Here's how the part is built. I have some questions about the finished solid (model axes, mm). Round coordinates to 2 decimals unless told otherwise and drop trailing zeros. Order: outer loops, then holes, each group sorted by start corner. A loop starts at its lowest first (then second) coordinate and runs counter-clockwise, first axis right, second up. Notation, with made-up numbers: (9.5, 5) - (27.5, 5) arc R9 cw to (27.5, 18) - close; hole circle Ø11 at (-25.5, 57.5). An arc over 180 degrees is marked (long way). One line per item, written item: value.
Autodesk Inventor part; units mm, degrees
ref_plane "YZ Plane" through (0, 0, 0) normal (1, 0, 0) x (0, 1, 0)
ref_plane "XZ Plane" through (0, 0, 0) normal (0, 1, 0) x (-1, 0, 0)
ref_plane "XY Plane" through (0, 0, 0) normal (0, 0, 1) x (1, 0, 0)
sketch "Sketch1" plane through (0, 0, 0) normal (0, 0, 1) x (1, 0, 0)
  circle A0 centre (13.2036, 20.3187) radius 2.0955
  circle A1 centre (-12.1964, 20.3187) radius 2.0955
  line L0 (4.3471, -17.7813) -> (-3.3398, -17.7813)
  arc A2 (4.3471, -17.7813) -> (7.3873, -15.5216) centre (4.3471, -14.6063) ccw
  arc A3 (-6.38, -15.5216) -> (-3.3398, -17.7813) centre (-3.3398, -14.6063) ccw
  line L1 (-16.7567, 18.9458) -> (-6.38, -15.5216)
  line L2 (17.764, 18.9458) -> (7.3873, -15.5216)
  arc A4 (-12.1964, 25.0812) -> (-16.7567, 18.9458) centre (-12.1964, 20.3187) ccw
  arc A5 (17.764, 18.9458) -> (13.2036, 25.0812) centre (13.2036, 20.3187) ccw
  line L3 (-12.1964, 25.0812) -> (13.2036, 25.0812)
  point P0 (0, 0)
  point P1 (-12.1964, 25.0812)
  point P2 (17.4758, 18.214)
  point P3 (-16.4686, 18.214)
  dimension "d1" = 3.175
  dimension "d8" = 4.191
  dimension "d9" = 4.191
  dimension "d25" = 9.525
  dimension "d26" = 9.525
extrude "Extrusion1" add sketch "Sketch1" along normal blind 1.5875
equation "\"BendRadius\" = Thickness"
equation "\"BendReliefWidth\" = Thickness"
equation "\"BendReliefDepth\" = 0.5 * Thickness"
equation "\"CornerReliefSize\" = 4 * Thickness"
equation "\"MinimumRemnant\" = 2 * Thickness"
equation "\"TransitionRadius\" = BendRadius"
equation "\"JacobiRadiusSize\" = BendRadius"
equation "\"GapSize\" = Thickness"
properties part number "Hook Gussett" material "Acetal Resin, White"
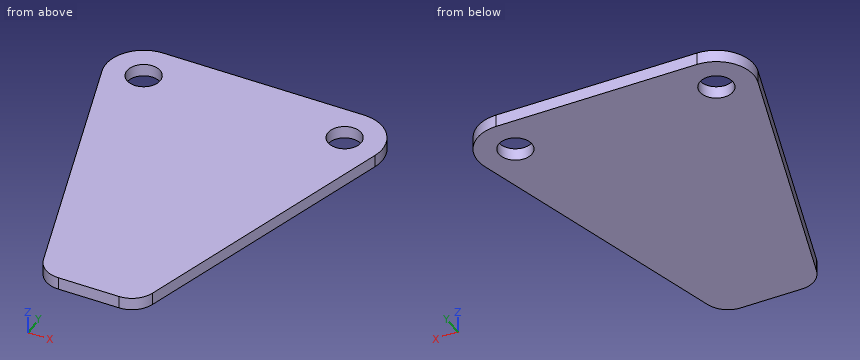
Q1. Will this pin go through, and if not, where does the flat tip stop? pin 1 (3.5 mm diameter, centred on x = 13.2, y = 20.32, fed in from -Z).
Results list:
pin 1: through
Q2. If we section it at A-A, the plane z = 0.35: Please give me the cut outline in (x, y) (1 decimal).
Results list:
outline: (-16.8, 18.9) - (-6.4, -15.5) arc R3.2 ccw to (-3.3, -17.8) - (4.3, -17.8) arc R3.2 ccw to (7.4, -15.5) - (17.8, 18.9) arc R4.8 ccw to (13.2, 25.1) - (-12.2, 25.1) arc R4.8 ccw to start; hole circle Ø4.2 at (-12.2, 20.3); hole circle Ø4.2 at (13.2, 20.3)
Q3. If we section it at C-C, the plane x = -9: Please give me the cut outline in (y, z), then the cut area to 3 significant figures.
Results list:
outline: (-6.82, 0) - (25.08, 0) - (25.08, 1.59) - (-6.82, 1.59) - close
area: 50.6 mm²
Q4. If I drill on line 1 along X through (y, z) = (12, 0.4); line 2 along X through (y, z) = (3, 1.2), over which ranges is the centre line in solid material (lowest first)?
Results list:
line 1: -14.67 to 15.67
line 2: -11.96 to 12.96
Q5. If we section it at B-B, the plane y = -5: Please give me the cut outline in (x, z), then the cut area to 3 significant figures.
Results list:
outline: (-9.55, 0) - (10.55, 0) - (10.55, 1.59) - (-9.55, 1.59) - close
area: 31.9 mm²
